from build123d import *

# Parameters (mm, degrees)
SKETCH1_W                      = 74
SKETCH1_H                      = 56
BOSS_EXTRUDE1_DEPTH            = 10
BOSS_EXTRUDE2_DEPTH            = 10
BOSS_EXTRUDE3_START            = 10
BOSS_EXTRUDE3_DEPTH            = 10
BOSS_EXTRUDE4_DEPTH            = 10
SKETCH5_R                      = 20
BOSS_EXTRUDE5_DEPTH            = 40
SKETCH6_R                      = 15
BOSS_EXTRUDE6_DEPTH            = 100
CUT_EXTRUDE1_START             = -60
CUT_EXTRUDE1_DEPTH             = 60
F_10_0_10_DIAMETER_HOLE1_D     = 10
F_10_0_10_DIAMETER_HOLE1_DEPTH = 10
F_10_0_10_DIAMETER_HOLE2_D     = 10
F_10_0_10_DIAMETER_HOLE2_DEPTH = 76
CHAMFER1_SIZE                  = 2


with BuildPart() as part:
    # Sketch1 → Boss-Extrude1 (new body)
    with BuildSketch(Plane.XY):
        Rectangle(SKETCH1_W, SKETCH1_H)
    extrude(amount=-BOSS_EXTRUDE1_DEPTH)

    # Sketch2 → Boss-Extrude2 (add)
    with BuildSketch(Plane.XZ.offset(28)):
        with BuildLine():
            Line((-37, 0), (37, 0))
            Line((37, 0), (37, -10))
            Line((37, -10), (13.060137394, -52.377859531))
            ThreePointArc((13.060137394, -52.377859531), (0, -60), (-13.060137394, -52.377859531))
            Line((-13.060137394, -52.377859531), (-37, -10))
            Line((-37, -10), (-37, 0))
        make_face()
    extrude(amount=BOSS_EXTRUDE2_DEPTH)

    # Sketch3 → Boss-Extrude3 (add)
    with BuildSketch(Plane(origin=(0, 28, 0), x_dir=(-1, 0, 0), z_dir=(0, 1, 0)).offset(BOSS_EXTRUDE3_START)):
        with BuildLine():
            Line((-37, 0), (37, 0))
            Line((37, 0), (37, -10))
            Line((37, -10), (13.060137394, -52.377859531))
            ThreePointArc((13.060137394, -52.377859531), (0, -60), (-13.060137394, -52.377859531))
            Line((-13.060137394, -52.377859531), (-37, -10))
            Line((-37, -10), (-37, 0))
        make_face()
    extrude(amount=-BOSS_EXTRUDE3_DEPTH)

    # Sketch4 → Boss-Extrude4 (add)
    with BuildSketch(Plane.XY):
        with BuildLine():
            Line((18, -24), (-18, -24))
            ThreePointArc((-18, -24), (-30, 0), (-18, 24))
            Line((-18, 24), (18, 24))
            ThreePointArc((18, 24), (30, 0), (18, -24))
        make_face()
    extrude(amount=BOSS_EXTRUDE4_DEPTH)

    # Sketch5 → Boss-Extrude5 (add)
    with BuildSketch(Plane.XY.offset(10)):
        Circle(SKETCH5_R)
    extrude(amount=BOSS_EXTRUDE5_DEPTH)

    # Sketch6 → Boss-Extrude6 (add)
    with BuildSketch(Plane.XY.offset(50)):
        with Locations(Location((0, 0, 0), (0, 0, 180))):
            Circle(SKETCH6_R)
    extrude(amount=BOSS_EXTRUDE6_DEPTH)

    # Sketch7 → Cut-Extrude1 (cut)
    with BuildSketch(Plane.XY.offset(150).offset(CUT_EXTRUDE1_START)):
        with BuildLine():
            Line((-12.68857754, 8), (12.68857754, 8))
            ThreePointArc((12.68857754, 8), (0, 15), (-12.68857754, 8))
        make_face()
    extrude(amount=CUT_EXTRUDE1_DEPTH, mode=Mode.SUBTRACT)

    # Ø10.0 (10) Diameter Hole1
    with Locations(Plane(origin=(0, -38, 0), x_dir=(-1, 0, 0), z_dir=(0, -1, 0))):
        with Locations((0, 45)):
            Hole(F_10_0_10_DIAMETER_HOLE1_D / 2, depth=F_10_0_10_DIAMETER_HOLE1_DEPTH)

    # Ø10.0 (10) Diameter Hole2
    with Locations(Plane(origin=(0, 38, 0), x_dir=(1, 0, 0), z_dir=(0, 1, 0))):
        with Locations((0, 45)):
            Hole(F_10_0_10_DIAMETER_HOLE2_D / 2, depth=F_10_0_10_DIAMETER_HOLE2_DEPTH)

    # Chamfer1
    chamfer1_edges = [part.edges().sort_by_distance(p)[0] for p in [
        (4.163612428, -14.410563193, 150),
    ]]
    chamfer(chamfer1_edges, length=CHAMFER1_SIZE)


solid = part.part
Could you check a few things on this model? Use its own coordinates, in mm. A direction names the side the tool comes from. Round coordinates to 2 decimals unless told otherwise and drop trailing zeros. Order: outer loops, then holes, each group sorted by start corner. A loop starts at its lowest first (then second) coordinate and runs counter-clockwise, first axis right, second up. Notation, with made-up numbers: M 79.5,-24.75 L 100.5,-24.75 A29 ccw 100.5,9.25 Z; hole C -0.5,-36.75 d9. An arc over 180 degrees is marked long. One line per item, written item: value.
(1) Imagine slicing it at B-B (z = -15.5). Write out the boundary of the cut face in (x, y).
Ans:
outline: M -33.89,-38 L 33.89,-38 L 33.89,-28 L -33.89,-28 Z; M -33.89,28 L 33.89,28 L 33.89,38 L -33.89,38 Z
(2) Imagine slicing it at C-C (z = -45). Write out the boundary of the cut face in (x, y), and give its area (3 significant figures).
Ans:
outline: M -17.23,-38 L -5,-38 L -5,-28 L -17.23,-28 Z; M -17.23,28 L -5,28 L -5,38 L -17.23,38 Z; M 5,-38 L 17.23,-38 L 17.23,-28 L 5,-28 Z; M 5,28 L 17.23,28 L 17.23,38 L 5,38 Z
area: 489 mm^2
(3) I need wall thicknesses on line 1 along Z through (x, y) = (0, 32.75); line 2 along X through (y, z) = (34, -45); line 3 along Z through (x, y) = (23.5, -9). Which ranges of each line are inside material? Lowest first, please. Write a range as from..to.
Ans:
line 1: z = -60..-50, -40..0
line 2: x = -17.23..-5, 5..17.23
line 3: z = -10..10
(4) If we mould it in two halves opening along Z, with no side actions, what happens to faces 1 (the conical face through (-0.416, -13.313, 149.681)), 2 (the cylindrical face through (0.651, 32.93, -49.957)), 3 (the cylindrical face through (-30, 0, 5))? For each: released by +Z, released by -Z, zero draft, split by the parting line, or undercut.
Ans:
face 1: released by +Z
face 2: undercut
face 3: zero draft
(5) I'm going to push flat-ended pins straight in: P1, Ø5, axis at x = 7.5, z = 3.5, coming from the -Y side; P2, Ø5, axis at x = -23, y = -18, coming from the +Z side; P3, Ø3, axis at x = 15, y = 24.5, coming from the -Z side. Where does each tip first touch, or does it pass through?
Ans:
P1: stops at y = -24
P2: stops at z = 10
P3: stops at z = -10
(6) Imagine slicing it at D-D (x = 33.5). Write out the boundary of the cut face in (y, z), and give its area (3 significant figures).
Ans:
outline: M -38,-16.2 L -28,-16.2 L -28,-10 L 28,-10 L 28,-16.2 L 38,-16.2 L 38,0 L -38,0 Z
area: 884 mm^2
(7) Which directions (+Z, -Z, +X, -X, +Y, -Y) give clear straight access to the entire face, cutting with the end or side of a thin tool? Please do faces 4 (the flat face through (3, 15, 50)), 5 (the flat face through (1, -28, -29)), 6 (the flat face through (0, -24, 5)), 7 (the flat face through (0, 24, 5)).
Ans:
face 4: +Z
face 5: -Z, +X, -X
face 6: +Z, +X, -X, -Y
face 7: +Z, +X, -X, +Y
(8) Imagine slicing it at A-A (x = 0). Count the separate pieces of the cut face and the enclosed holes in it, and give its area (3 significant figures).
Ans:
separate pieces: 3
enclosed holes: 0
area: 6,220 mm^2
